Work out the finished part from the listing and answer in its coordinate system (mm). Face numbers are marked on the shaded views. A direction names the side the tool comes from. Coordinates: 2 decimals unless noted, no trailing zeros. Order: outer loops, then holes, each group sorted by start corner. A loop starts at its lowest first (then second) coordinate and runs counter-clockwise, first axis right, second up.
```python
from build123d import *

# Parameters (mm, degrees)
EXTRUDE1_DEPTH = 6.73
SKETCH4_R      = 1.545336663
EXTRUDE2_DEPTH = 9.295442022
CHAMFER1_SIZE  = 0.525


with BuildPart() as part:
    # Sketch1 → Extrude1 (new body)
    with BuildSketch(Plane(origin=(0, 0, 0), x_dir=(1, 0, 0), z_dir=(0, 1, 0))):
        Polygon((0, 3.666174209), (-3.175, 1.833087105), (-3.175, -1.833087105), (0, -3.666174209), (3.175, -1.833087105), (3.175, 1.833087105), align=None)
    extrude(amount=-EXTRUDE1_DEPTH)

    # Sketch4 → Extrude2 (cut, through all)
    with BuildSketch(Plane(origin=(0, 0, 0), x_dir=(-1, 0, 0), z_dir=(0, 1, 0))):
        with Locations(Location((0, 0, 0), (0, 0, 90))):
            Circle(SKETCH4_R)
    extrude(amount=-EXTRUDE2_DEPTH, mode=Mode.SUBTRACT)

    # Chamfer1
    chamfer1_edges = [part.edges().sort_by_distance(p)[0] for p in [
        (0, -6.73, -1.545336663),
        (0, 0, -1.545336663),
    ]]
    chamfer(chamfer1_edges, length=CHAMFER1_SIZE)

    # Sketch5 → Cut-Revolve1 (revolve, cut)
    with BuildSketch(Plane.XY):
        Polygon((-3.16, -6.73), (-3.666174209, -6.73), (-4.172348419, -6.73), (-4.172348419, 0), (-3.666174209, 0), (-3.666174209, -0.560833333), (-3.16, -0.560833333), (-3.16, -1.402083333), (-3.651490136, -1.402083333), (-3.645798403, -1.728162487), (-3.16, -2.421954508), (-3.16, -2.748083333), (-3.627995619, -2.748083333), (-3.622303886, -3.074162487), (-3.16, -3.73440086), (-3.16, -4.060529685), (-3.605086782, -4.060529685), (-3.59939505, -4.386608839), (-3.16, -5.014130003), (-3.16, -5.340258828), (-3.582749027, -5.340258828), (-3.577057294, -5.666337982), (-3.16, -6.261957525), align=None)
    revolve(axis=Axis((0, 0, 0), (0, -1, 0)), mode=Mode.SUBTRACT)


solid = part.part
```
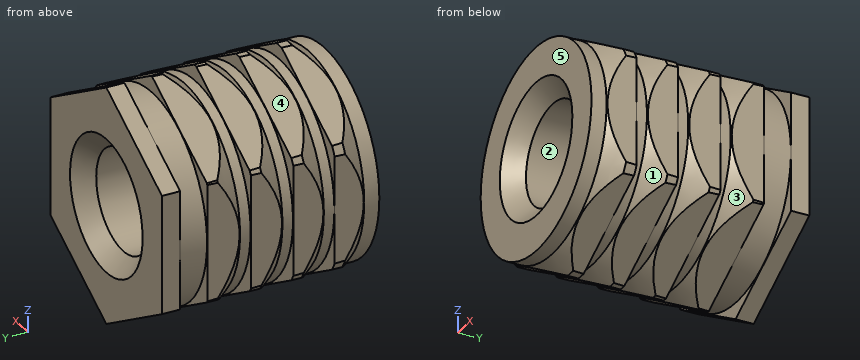
1. The mould has two halves that part along Y. Classify the marked faces 3, 4 and 5: released by +Y, released by -Y, zero draft, split by the parting line, or undercut.
2. The part is cut by section B-B (y = -3.5). Determine the outline of the cut face in (x, z) (3 decimals), plus the area to 3 significant figures.
3. For the marked faces 1 and 2, determine the directions among +Z, -Z, +X, -X, +Y, -Y from which every point of the face is accessible in a straight line to the end or side of a thin tool.
4. The part is cut by section A-A (y = -4.25). Determine the outline of the cut face in (x, z) (3 decimals), plus the area to 3 significant figures.
5. Consider probe 1 along X at (y, z) = (-3.5, 0) (3 decimals); probe 2 along Y at (x, z) = (2.5, -2); probe 3 along Y at (x, z) = (0, -3.5). Determine where each line is inside the solid, lowest interval first.
Worked out:
1. face 3: undercut
1. face 4: zero draft
1. face 5: released by -Y
2. outline: (-3.175, -0.984) arc R3.324 ccw to (-2.44, -2.257) - (-0.735, -3.242) arc R3.324 ccw to (0.735, -3.242) - (2.44, -2.257) arc R3.324 ccw to (3.175, -0.984) - (3.175, 0.984) arc R3.324 ccw to (2.44, 2.257) - (0.735, 3.242) arc R3.324 ccw to (-0.735, 3.242) - (-2.44, 2.257) arc R3.324 ccw to (-3.175, 0.984) - close; hole circle Ø3.091 at (0, 0)
2. area: 26.0 mm2
3. face 1: none
3. face 2: +Y, -Y
4. outline: (-3.175, -1.701) arc R3.602 ccw to (-3.06, -1.899) - (-0.115, -3.6) arc R3.602 ccw to (0.115, -3.6) - (3.06, -1.899) arc R3.602 ccw to (3.175, -1.701) - (3.175, 1.701) arc R3.602 ccw to (3.06, 1.899) - (0.115, 3.6) arc R3.602 ccw to (-0.115, 3.6) - (-3.06, 1.899) arc R3.602 ccw to (-3.175, 1.701) - close; hole circle Ø3.091 at (0, 0)
4. area: 27.4 mm2
5. probe 1: x = -3.175 to -1.545, 1.545 to 3.175
5. probe 2: y = -6.2 to -5.34, -4.95 to -4.06, -3.68 to -2.75, -2.36 to -1.4, -0.56 to 0
5. probe 3: y = -5.78 to -5.34, -4.53 to -4.06, -3.25 to -2.75, -1.94 to -1.4, -0.56 to 0
